Here's how the part is built. I have some questions about the finished solid (model axes, mm). Face numbers are marked on the shaded views. A direction names the side the tool comes from. Give positions to 0.01 mm unless a question says otherwise; leave off trailing zeros. Loops run counter-clockwise (first coordinate to the right, second up) from the corner with the lowest first, then second, coordinate; pieces in that order, holes last. Notation, with made-up numbers: (40.25, -10) - (53.25, -10) arc R13 cw to (53.25, 14) - close; hole circle Ø7 at (67, 55.25). An arc over 180 degrees is marked (long way). One line per item, written item: value. Start each with the question number.
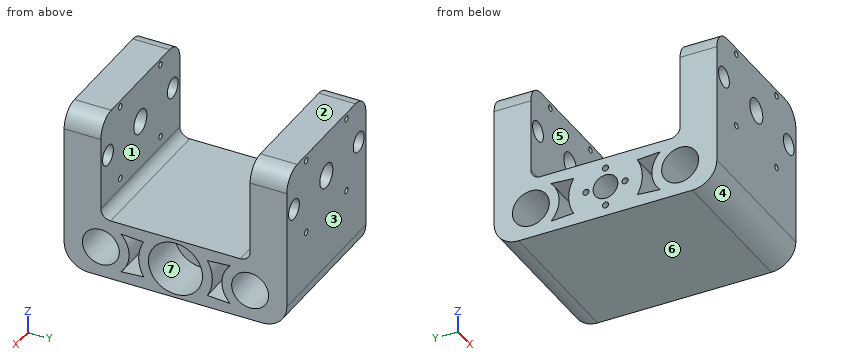
```python
from build123d import *

# Parameters (mm, degrees)
SKETCH1_R                      = 5.05
SKETCH1_R_2                    = 7.55
BOSS_EXTRUDE1_DEPTH            = 30.5
CUT_EXTRUDE1_REACH             = 47.5
SKETCH2_R                      = 5
SKETCH2_R_2                    = 4.15
SKETCH2_R_3                    = 1.25
CUT_EXTRUDE1_DIRECTION_2_REACH = 47.5
CROQUIS4_W                     = 42
CROQUIS4_H                     = 61
CORTAR_EXTRUIR1_DEPTH          = 62
REDONDEO4_R                    = 4
REDONDEO5_R                    = 8
CROQUIS5_R                     = 11.05
CORTAR_EXTRUIR2_DEPTH          = 20
CROQUIS6_R                     = 1.25
CORTAR_EXTRUIR3_DEPTH          = 42
CORTAR_EXTRUIR4_DEPTH          = 61


with BuildPart() as part:
    # Sketch1 → Boss-Extrude1 (new body, symmetric)
    with BuildSketch(Plane(origin=(0, 0, 0), x_dir=(0, 0, -1), z_dir=(1, 0, 0))):
        with BuildLine():
            Line((0, 15.5), (0, -15.5))
            Line((0, -15.5), (-42, -15.5))
            Line((-42, -15.5), (-42, -45.5))
            Line((-42, -45.5), (15, -45.5))
            ThreePointArc((15, -45.5), (22.071067812, -42.571067812), (25, -35.5))
            Line((25, -35.5), (25, 35.5))
            ThreePointArc((25, 35.5), (22.071067812, 42.571067812), (15, 45.5))
            Line((15, 45.5), (-42, 45.5))
            Line((-42, 45.5), (-42, 15.5))
            Line((-42, 15.5), (0, 15.5))
        make_face()
        with Locations(Location((12.5, 0, 0), (0, 0, 180))):  # turned: the seam where the file's is
            Circle(SKETCH1_R, mode=Mode.SUBTRACT)
        with Locations((12.5, 30.5)):
            Circle(SKETCH1_R_2, mode=Mode.SUBTRACT)
        with Locations(Location((12.5, -30.5, 0), (0, 0, 180))):  # turned: the seam where the file's is
            Circle(SKETCH1_R_2, mode=Mode.SUBTRACT)
    extrude(amount=BOSS_EXTRUDE1_DEPTH, both=True)

    # Cut-Extrude1: up to this face of the body (flat: up to its plane)
    cut_extrude1_end = Plane(part.part.faces().sort_by_distance((0, 45.5, 13.5))[0])
    # Sketch2 → Cut-Extrude1 (cut, up to the picked face)
    with BuildSketch(Plane(origin=(0, 0, 0), x_dir=(1, 0, 0), z_dir=(0, 1, 0)), mode=Mode.PRIVATE) as cut_extrude1_sk1:
        with Locations(Location((0, -24, 0), (0, 0, 90))):  # turned: the seam where the file's is
            Circle(SKETCH2_R)
    cut_extrude1_tool1 = split(extrude(cut_extrude1_sk1.sketch, amount=CUT_EXTRUDE1_REACH, mode=Mode.PRIVATE), bisect_by=cut_extrude1_end, keep=Keep.BOTH, mode=Mode.PRIVATE)
    add(cut_extrude1_tool1.solids().sort_by(Axis((0, 0, 24), (0, 1, 0)))[0], mode=Mode.SUBTRACT)
    # Sketch2 → Cut-Extrude1 (cut, up to the picked face)
    with BuildSketch(Plane(origin=(0, 0, 0), x_dir=(1, 0, 0), z_dir=(0, 1, 0)), mode=Mode.PRIVATE) as cut_extrude1_sk2:
        with Locations(Location((25, -24, 0), (0, 0, 90))):  # turned: the seam where the file's is
            Circle(SKETCH2_R_2)
    cut_extrude1_tool2 = split(extrude(cut_extrude1_sk2.sketch, amount=CUT_EXTRUDE1_REACH, mode=Mode.PRIVATE), bisect_by=cut_extrude1_end, keep=Keep.BOTH, mode=Mode.PRIVATE)
    add(cut_extrude1_tool2.solids().sort_by(Axis((25, 0, 24), (0, 1, 0)))[0], mode=Mode.SUBTRACT)
    # Sketch2 → Cut-Extrude1 (cut, up to the picked face)
    with BuildSketch(Plane(origin=(0, 0, 0), x_dir=(1, 0, 0), z_dir=(0, 1, 0)), mode=Mode.PRIVATE) as cut_extrude1_sk3:
        with Locations(Location((-25, -24, 0), (0, 0, 90))):  # turned: the seam where the file's is
            Circle(SKETCH2_R_2)
    cut_extrude1_tool3 = split(extrude(cut_extrude1_sk3.sketch, amount=CUT_EXTRUDE1_REACH, mode=Mode.PRIVATE), bisect_by=cut_extrude1_end, keep=Keep.BOTH, mode=Mode.PRIVATE)
    add(cut_extrude1_tool3.solids().sort_by(Axis((-25, 0, 24), (0, 1, 0)))[0], mode=Mode.SUBTRACT)
    # Sketch2 → Cut-Extrude1 (cut, up to the picked face)
    with BuildSketch(Plane(origin=(0, 0, 0), x_dir=(1, 0, 0), z_dir=(0, 1, 0)), mode=Mode.PRIVATE) as cut_extrude1_sk4:
        with Locations(Location((15.5, -39.5, 0), (0, 0, 90))):  # turned: the seam where the file's is
            Circle(SKETCH2_R_3)
    cut_extrude1_tool4 = split(extrude(cut_extrude1_sk4.sketch, amount=CUT_EXTRUDE1_REACH, mode=Mode.PRIVATE), bisect_by=cut_extrude1_end, keep=Keep.BOTH, mode=Mode.PRIVATE)
    add(cut_extrude1_tool4.solids().sort_by(Axis((15.5, 0, 39.5), (0, 1, 0)))[0], mode=Mode.SUBTRACT)
    # Sketch2 → Cut-Extrude1 (cut, up to the picked face)
    with BuildSketch(Plane(origin=(0, 0, 0), x_dir=(1, 0, 0), z_dir=(0, 1, 0)), mode=Mode.PRIVATE) as cut_extrude1_sk5:
        with Locations(Location((-15.5, -39.5, 0), (0, 0, 90))):  # turned: the seam where the file's is
            Circle(SKETCH2_R_3)
    cut_extrude1_tool5 = split(extrude(cut_extrude1_sk5.sketch, amount=CUT_EXTRUDE1_REACH, mode=Mode.PRIVATE), bisect_by=cut_extrude1_end, keep=Keep.BOTH, mode=Mode.PRIVATE)
    add(cut_extrude1_tool5.solids().sort_by(Axis((-15.5, 0, 39.5), (0, 1, 0)))[0], mode=Mode.SUBTRACT)
    # Sketch2 → Cut-Extrude1 (cut, up to the picked face)
    with BuildSketch(Plane(origin=(0, 0, 0), x_dir=(1, 0, 0), z_dir=(0, 1, 0)), mode=Mode.PRIVATE) as cut_extrude1_sk6:
        with Locations(Location((-15.5, -8.5, 0), (0, 0, 90))):  # turned: the seam where the file's is
            Circle(SKETCH2_R_3)
    cut_extrude1_tool6 = split(extrude(cut_extrude1_sk6.sketch, amount=CUT_EXTRUDE1_REACH, mode=Mode.PRIVATE), bisect_by=cut_extrude1_end, keep=Keep.BOTH, mode=Mode.PRIVATE)
    add(cut_extrude1_tool6.solids().sort_by(Axis((-15.5, 0, 8.5), (0, 1, 0)))[0], mode=Mode.SUBTRACT)
    # Sketch2 → Cut-Extrude1 (cut, up to the picked face)
    with BuildSketch(Plane(origin=(0, 0, 0), x_dir=(1, 0, 0), z_dir=(0, 1, 0)), mode=Mode.PRIVATE) as cut_extrude1_sk7:
        with Locations(Location((15.5, -8.5, 0), (0, 0, 90))):  # turned: the seam where the file's is
            Circle(SKETCH2_R_3)
    cut_extrude1_tool7 = split(extrude(cut_extrude1_sk7.sketch, amount=CUT_EXTRUDE1_REACH, mode=Mode.PRIVATE), bisect_by=cut_extrude1_end, keep=Keep.BOTH, mode=Mode.PRIVATE)
    add(cut_extrude1_tool7.solids().sort_by(Axis((15.5, 0, 8.5), (0, 1, 0)))[0], mode=Mode.SUBTRACT)

    # Cut-Extrude1 direction 2: up to this face of the body (flat: up to its plane)
    cut_extrude1_direction_2_end = Plane(part.part.faces().sort_by_distance((0, -45.5, 13.5))[0])
    # Sketch2 → Cut-Extrude1 direction 2 (cut, up to the picked face)
    with BuildSketch(Plane(origin=(0, 0, 0), x_dir=(1, 0, 0), z_dir=(0, 1, 0)), mode=Mode.PRIVATE) as cut_extrude1_direction_2_sk1:
        with Locations(Location((0, -24, 0), (0, 0, 90))):  # turned: the seam where the file's is
            Circle(SKETCH2_R)
    cut_extrude1_direction_2_tool1 = split(extrude(cut_extrude1_direction_2_sk1.sketch, amount=-CUT_EXTRUDE1_DIRECTION_2_REACH, mode=Mode.PRIVATE), bisect_by=cut_extrude1_direction_2_end, keep=Keep.BOTH, mode=Mode.PRIVATE)
    add(cut_extrude1_direction_2_tool1.solids().sort_by(Axis((0, 0, 24), (0, -1, 0)))[0], mode=Mode.SUBTRACT)
    # Sketch2 → Cut-Extrude1 direction 2 (cut, up to the picked face)
    with BuildSketch(Plane(origin=(0, 0, 0), x_dir=(1, 0, 0), z_dir=(0, 1, 0)), mode=Mode.PRIVATE) as cut_extrude1_direction_2_sk2:
        with Locations(Location((25, -24, 0), (0, 0, 90))):  # turned: the seam where the file's is
            Circle(SKETCH2_R_2)
    cut_extrude1_direction_2_tool2 = split(extrude(cut_extrude1_direction_2_sk2.sketch, amount=-CUT_EXTRUDE1_DIRECTION_2_REACH, mode=Mode.PRIVATE), bisect_by=cut_extrude1_direction_2_end, keep=Keep.BOTH, mode=Mode.PRIVATE)
    add(cut_extrude1_direction_2_tool2.solids().sort_by(Axis((25, 0, 24), (0, -1, 0)))[0], mode=Mode.SUBTRACT)
    # Sketch2 → Cut-Extrude1 direction 2 (cut, up to the picked face)
    with BuildSketch(Plane(origin=(0, 0, 0), x_dir=(1, 0, 0), z_dir=(0, 1, 0)), mode=Mode.PRIVATE) as cut_extrude1_direction_2_sk3:
        with Locations(Location((-25, -24, 0), (0, 0, 90))):  # turned: the seam where the file's is
            Circle(SKETCH2_R_2)
    cut_extrude1_direction_2_tool3 = split(extrude(cut_extrude1_direction_2_sk3.sketch, amount=-CUT_EXTRUDE1_DIRECTION_2_REACH, mode=Mode.PRIVATE), bisect_by=cut_extrude1_direction_2_end, keep=Keep.BOTH, mode=Mode.PRIVATE)
    add(cut_extrude1_direction_2_tool3.solids().sort_by(Axis((-25, 0, 24), (0, -1, 0)))[0], mode=Mode.SUBTRACT)
    # Sketch2 → Cut-Extrude1 direction 2 (cut, up to the picked face)
    with BuildSketch(Plane(origin=(0, 0, 0), x_dir=(1, 0, 0), z_dir=(0, 1, 0)), mode=Mode.PRIVATE) as cut_extrude1_direction_2_sk4:
        with Locations(Location((15.5, -39.5, 0), (0, 0, 90))):  # turned: the seam where the file's is
            Circle(SKETCH2_R_3)
    cut_extrude1_direction_2_tool4 = split(extrude(cut_extrude1_direction_2_sk4.sketch, amount=-CUT_EXTRUDE1_DIRECTION_2_REACH, mode=Mode.PRIVATE), bisect_by=cut_extrude1_direction_2_end, keep=Keep.BOTH, mode=Mode.PRIVATE)
    add(cut_extrude1_direction_2_tool4.solids().sort_by(Axis((15.5, 0, 39.5), (0, -1, 0)))[0], mode=Mode.SUBTRACT)
    # Sketch2 → Cut-Extrude1 direction 2 (cut, up to the picked face)
    with BuildSketch(Plane(origin=(0, 0, 0), x_dir=(1, 0, 0), z_dir=(0, 1, 0)), mode=Mode.PRIVATE) as cut_extrude1_direction_2_sk5:
        with Locations(Location((-15.5, -39.5, 0), (0, 0, 90))):  # turned: the seam where the file's is
            Circle(SKETCH2_R_3)
    cut_extrude1_direction_2_tool5 = split(extrude(cut_extrude1_direction_2_sk5.sketch, amount=-CUT_EXTRUDE1_DIRECTION_2_REACH, mode=Mode.PRIVATE), bisect_by=cut_extrude1_direction_2_end, keep=Keep.BOTH, mode=Mode.PRIVATE)
    add(cut_extrude1_direction_2_tool5.solids().sort_by(Axis((-15.5, 0, 39.5), (0, -1, 0)))[0], mode=Mode.SUBTRACT)
    # Sketch2 → Cut-Extrude1 direction 2 (cut, up to the picked face)
    with BuildSketch(Plane(origin=(0, 0, 0), x_dir=(1, 0, 0), z_dir=(0, 1, 0)), mode=Mode.PRIVATE) as cut_extrude1_direction_2_sk6:
        with Locations(Location((-15.5, -8.5, 0), (0, 0, 90))):  # turned: the seam where the file's is
            Circle(SKETCH2_R_3)
    cut_extrude1_direction_2_tool6 = split(extrude(cut_extrude1_direction_2_sk6.sketch, amount=-CUT_EXTRUDE1_DIRECTION_2_REACH, mode=Mode.PRIVATE), bisect_by=cut_extrude1_direction_2_end, keep=Keep.BOTH, mode=Mode.PRIVATE)
    add(cut_extrude1_direction_2_tool6.solids().sort_by(Axis((-15.5, 0, 8.5), (0, -1, 0)))[0], mode=Mode.SUBTRACT)
    # Sketch2 → Cut-Extrude1 direction 2 (cut, up to the picked face)
    with BuildSketch(Plane(origin=(0, 0, 0), x_dir=(1, 0, 0), z_dir=(0, 1, 0)), mode=Mode.PRIVATE) as cut_extrude1_direction_2_sk7:
        with Locations(Location((15.5, -8.5, 0), (0, 0, 90))):  # turned: the seam where the file's is
            Circle(SKETCH2_R_3)
    cut_extrude1_direction_2_tool7 = split(extrude(cut_extrude1_direction_2_sk7.sketch, amount=-CUT_EXTRUDE1_DIRECTION_2_REACH, mode=Mode.PRIVATE), bisect_by=cut_extrude1_direction_2_end, keep=Keep.BOTH, mode=Mode.PRIVATE)
    add(cut_extrude1_direction_2_tool7.solids().sort_by(Axis((15.5, 0, 8.5), (0, -1, 0)))[0], mode=Mode.SUBTRACT)

    # Croquis4 → Cortar-Extruir1 (cut, through all)
    with BuildSketch(Plane(origin=(30.5, 0, 0), x_dir=(0, 0, -1), z_dir=(1, 0, 0))):
        with Locations((-21, 0)):
            Rectangle(CROQUIS4_W, CROQUIS4_H)
    extrude(amount=-CORTAR_EXTRUIR1_DEPTH, mode=Mode.SUBTRACT)

    # Redondeo4
    redondeo4_edges = [part.edges().sort_by_distance(p)[0] for p in [
        (0, 30.5, 0),
        (0, -30.5, 0),
    ]]
    fillet(redondeo4_edges, radius=REDONDEO4_R)

    # Redondeo5
    redondeo5_edges = [part.edges().sort_by_distance(p)[0] for p in [
        (-30.5, 38, 42),
        (-30.5, -38, 42),
        (30.5, -38, 42),
        (30.5, 38, 42),
    ]]
    fillet(redondeo5_edges, radius=REDONDEO5_R)

    # Croquis5 → Cortar-Extruir2 (cut)
    with BuildSketch(Plane(origin=(30.5, 0, 0), x_dir=(0, 0, -1), z_dir=(1, 0, 0))):
        with Locations((12.5, 0)):
            Circle(CROQUIS5_R)
    extrude(amount=-CORTAR_EXTRUIR2_DEPTH, mode=Mode.SUBTRACT)

    # Croquis6 → Cortar-Extruir3 (cut, through all)
    with BuildSketch(Plane(origin=(10.5, 0, 0), x_dir=(0, 0, -1), z_dir=(1, 0, 0))):
        with Locations((12.5, 8)):
            Circle(CROQUIS6_R)
        with Locations((20.5, 0)):
            Circle(CROQUIS6_R)
        with Locations((12.5, -8)):
            Circle(CROQUIS6_R)
        with Locations((4.5, 0)):
            Circle(CROQUIS6_R)
    extrude(amount=-CORTAR_EXTRUIR3_DEPTH, mode=Mode.SUBTRACT)

    # Croquis8 → Cortar-Extruir4 (cut)
    with BuildSketch(Plane(origin=(30.5, 0, 0), x_dir=(0, 0, -1), z_dir=(1, 0, 0))):
        with BuildLine():
            Line((4.332916677, 22.332916677), (4.975, 13.033682327))
            ThreePointArc((4.975, 13.033682327), (12.5, 15.05), (20.025, 13.033682327))
            Line((20.025, 13.033682327), (20.667083323, 22.332916677))
            ThreePointArc((20.667083323, 22.332916677), (12.5, 18.95), (4.332916677, 22.332916677))
        make_face()
        with BuildLine():
            Line((4.332916677, -22.332916677), (4.975, -13.033682327))
            ThreePointArc((4.975, -13.033682327), (12.5, -15.05), (20.025, -13.033682327))
            Line((20.025, -13.033682327), (20.667083323, -22.332916677))
            ThreePointArc((20.667083323, -22.332916677), (12.5, -18.95), (4.332916677, -22.332916677))
        make_face()
    extrude(amount=-CORTAR_EXTRUIR4_DEPTH, mode=Mode.SUBTRACT)


solid = part.part
```
(1) If we mould it in two halves opening along Y, with no side actions, what happens to the marked faces 1, 2, 3 and 4? For each: pulls with the +Y half, pulls with the -Y half, needs draft (parallel to the pull), parting line crosses it, or undercut.
(2) If we section it at A-A on z = 8.5: List the corners of the cut face in (x, y) for me, plus the area to 3 significant figures.
(3) For the marked faces 5, 6 and 7, which set-ups out of +Z, -Z, +X, -X, +Y, -Y let a thin tool reach every point of the face, with its end or its side?
(4) Please list where these lines run through material, in increasing order: probe 1 along X at (y, z) = (41, 24); probe 2 along Y at (x, z) = (-17, 19.5); probe 3 along Z at (x, y) = (-23, 37). Write a range as from..to.
(5) Will this pin go through, and if not, where does the flat tip stop? pin 1 (12 mm diameter, centred on x = -8.5, y = -12, fed in from +Z).
(6) If we section it at B-B on z = 24: Give the number of separate pieces and of enclosed holes in the cut face, plus the area to 3 significant figures.
(7) If we section it at C-C on y = 0: List the corners of the cut face in (x, z) for me.
Found:
1. face 1: undercut
1. face 2: needs draft
1. face 3: pulls with the +Y half
1. face 4: pulls with the -Y half
2. outline: (-30.5, -45.5) - (-16.75, -45.5) - (-16.75, -30.5) - (-30.5, -30.5) - close; (-30.5, 30.5) - (-16.75, 30.5) - (-16.75, 45.5) - (-30.5, 45.5) - close; (-14.25, -45.5) - (14.25, -45.5) - (14.25, -30.5) - (-14.25, -30.5) - close; (-14.25, 30.5) - (14.25, 30.5) - (14.25, 45.5) - (-14.25, 45.5) - close; (16.75, -45.5) - (30.5, -45.5) - (30.5, -30.5) - (16.75, -30.5) - close; (16.75, 30.5) - (30.5, 30.5) - (30.5, 45.5) - (16.75, 45.5) - close
2. area: 1,680 mm^2
3. face 5: +Z, +X, -X
3. face 6: -Z, +X, -X, +Y, -Y
3. face 7: +X
4. probe 1: -30.5..-29.15, -20.85..-5, 5..20.85, 29.15..30.5
4. probe 2: -45.5..-30.5, 30.5..45.5
4. probe 3: -24.89..-16.34, -8.66..20.36, 27.64..41.98
5. pin 1: z = 0
6. separate pieces: 8
6. enclosed holes: 0
6. area: 1,030 mm^2
7. outline: (-30.5, -25) - (30.5, -25) - (30.5, -23.55) - (10.5, -23.55) - (10.5, -21.75) - (-30.5, -21.75) - close; (-30.5, -19.25) - (10.5, -19.25) - (10.5, -17.55) - (-30.5, -17.55) - close; (-30.5, -7.45) - (10.5, -7.45) - (10.5, -5.75) - (-30.5, -5.75) - close; (-30.5, -3.25) - (10.5, -3.25) - (10.5, -1.45) - (30.5, -1.45) - (30.5, 0) - (-30.5, 0) - close
